from build123d import *

# Parameters (mm, degrees)
F0_W     = 100
F0_H     = 100
F1_DEPTH = 100
F3_DEPTH = 45


with BuildPart() as f1:
    # F0 (on Right) → F1 (new body)
    with BuildSketch(Plane.YZ):
        with Locations((50, 50)):
            Rectangle(F0_W, F0_H)
    extrude(amount=F1_DEPTH)

    # F2 (on face) → F3 (cut)
    with BuildSketch(Plane.XY.offset(100)):
        with BuildLine():
            ThreePointArc((10, 50), (2.928932, 52.928932), (0, 60))
            Line((0, 60), (0, 0))
            Line((0, 0), (25, 0))
            Line((25, 0), (25, 50))
            Line((25, 50), (10, 50))
        make_face()
        with BuildLine():
            Line((100, 0), (100, 60))
            ThreePointArc((100, 60), (97.071068, 52.928932), (90, 50))
            Line((90, 50), (75, 50))
            Line((75, 50), (75, 0))
            Line((75, 0), (100, 0))
        make_face()
    extrude(amount=-F3_DEPTH, mode=Mode.SUBTRACT)


solid = f1.part
Could you check a few things on this model? Use its own coordinates, in mm. A direction names the side the tool comes from. Coordinates: 2 decimals unless noted, no trailing zeros. Write each loop counter-clockwise with the first axis right and the second up, starting at its lowest first coordinate (ties: lowest second). Pieces come first, ordered by that corner, then holes. Notation, with made-up numbers: (-24, 60.25) - (20, 60.25) arc R7 cw to (20, 70.25) - close; hole circle Ø1 at (53, 21). An arc over 180 degrees is marked (long way). Put each result on its own line as item: value. Start each with the question number.
Q1. I'm going to push flat-ended pins straight in: P1, Ø22.5, axis at y = 19, z = 78, coming from the -X side; P2, Ø16.5, axis at x = 15.5, z = 69.5, coming from the -Y side; P3, Ø7.5, axis at x = 91.5, y = 39, coming from the +Z side. Where does each tip first touch, or does it pass through?
Q2. I want a section at A-A on z = 82. Write out the boundary of the cut face in (x, y).
Q3. Which directions (+Z, -Z, +X, -X, +Y, -Y) give clear straight access to the entire face, cutting with the end or side of a thin tool? Please do faces 1 (the flat face through (25, 25, 78)), 2 (the flat face through (83, 50, 78)), 3 (the flat face through (0, 60, 40)).
Q4. I want a section at B-B on y = 46.5. Write out the boundary of the cut face in (x, z), plus the area to 3 significant figures.
Q5. I want a section at C-C on x = 16.5. Write out the boundary of the cut face in (y, z).
Q6. Please list where these lines run through material, in increasing order: L1, parallel to X at y = 20.5, z = 58.5; L2, parallel to Y at x = 75.5, z = 63; L3, parallel to X at y = 53, z = 87.
Q7. I want a section at D-D on x = 92. Write out the boundary of the cut face in (y, z).
Checks:
1. P1: x = 25
1. P2: y = 50
1. P3: z = 55
2. outline: (0, 60) arc R10 ccw to (10, 50) - (25, 50) - (25, 0) - (75, 0) - (75, 50) - (90, 50) arc R10 ccw to (100, 60) - (100, 100) - (0, 100) - close
3. face 1: +Z, -X, -Y
3. face 2: +Z, +X, -Y
3. face 3: +Z, -Z, -X, +Y, -Y
4. outline: (0, 0) - (100, 0) - (100, 55) - (75, 55) - (75, 100) - (25, 100) - (25, 55) - (0, 55) - close
4. area: 7,750 mm²
5. outline: (0, 0) - (100, 0) - (100, 100) - (50, 100) - (50, 55) - (0, 55) - close
6. L1: 25 to 75
6. L2: 50 to 100
6. L3: 2.86 to 97.14
7. outline: (0, 0) - (100, 0) - (100, 100) - (50.2, 100) - (50.2, 55) - (0, 55) - close
